from build123d import *

# Parameters (mm, degrees)
SKETCH1_W                       = 69.85
SKETCH1_H                       = 25.4
BASE_FLANGE1_DEPTH              = 4.55422
F_7_32_0_21875_DIAMETER_HOLE1_D = 5.55625
BREAK_CORNER1_DEPTH             = 4.55422
SKETCH4_W                       = 34.925
SKETCH4_H                       = 3.175
TAB1_DEPTH                      = 4.55422
FILLET1_R                       = 9.525
CUT_EXTRUDE1_REACH              = 40.633
SKETCH7_R                       = 9.525
CUT_EXTRUDE3_DEPTH              = 2.38125
F_9_32_0_28125_DIAMETER_HOLE1_D = 7.14375
FILLET3_R                       = 12.7
CUT_EXTRUDE4_START              = -2.17297
CUT_EXTRUDE4_DEPTH              = 2.17297
CUT_EXTRUDE5_REACH              = 40.633


# Read off the part's stored shape, not the designer's step: Break-Corner1
# Sheet-metal steps are written as plain solids
with BuildPart() as part:
    # Sketch1 → Base-Flange1 (new body)
    with BuildSketch(Plane.XY):
        Rectangle(SKETCH1_W, SKETCH1_H)
    extrude(amount=BASE_FLANGE1_DEPTH)

    # 7/32 (0.21875) Diameter Hole1 (through all)
    with Locations(Plane.XY.offset(4.55422)):
        with Locations((-28.575, 6.35), (-28.575, -6.35), (28.575, 6.35), (28.575, -6.35)):
            Hole(F_7_32_0_21875_DIAMETER_HOLE1_D / 2)

    # Break-Corner1 outline → Break-Corner1 (cut)
    with BuildSketch(Plane.XY):
        with BuildLine():
            Line((34.925, -12.7), (34.925, -9.525))
            ThreePointArc((34.925, -9.525), (33.99506403, -11.77006403), (31.75, -12.7))
            Line((31.75, -12.7), (34.925, -12.7))
        make_face()
        with BuildLine():
            ThreePointArc((31.75, 12.7), (33.99506403, 11.77006403), (34.925, 9.525))
            Line((34.925, 9.525), (34.925, 12.7))
            Line((34.925, 12.7), (31.75, 12.7))
        make_face()
        with BuildLine():
            Line((-34.925, -12.7), (-31.75, -12.7))
            ThreePointArc((-31.75, -12.7), (-33.99506403, -11.77006403), (-34.925, -9.525))
            Line((-34.925, -9.525), (-34.925, -12.7))
        make_face()
        with BuildLine():
            ThreePointArc((-34.925, 9.525), (-33.99506403, 11.77006403), (-31.75, 12.7))
            Line((-31.75, 12.7), (-34.925, 12.7))
            Line((-34.925, 12.7), (-34.925, 9.525))
        make_face()
    extrude(amount=BREAK_CORNER1_DEPTH, mode=Mode.SUBTRACT)

    # Sketch4 → Tab1 (add)
    with BuildSketch(Plane(origin=(0, 0, 0), x_dir=(-1, 0, 0), z_dir=(0, 0, -1))):
        with Locations((0, -14.2875)):
            Rectangle(SKETCH4_W, SKETCH4_H)
    extrude(amount=-TAB1_DEPTH)

    # Fillet1
    # the kernel refuses this fillet: 9.525 mm, written as the material it adds along each edge
    with BuildSketch(Plane(origin=(-17.4625, -12.7, 0), x_dir=(-1, 0, 0), z_dir=(0, 0, 1))) as fillet1_piece_1:
        with BuildLine():
            CenterArc((7.099515829, 9.525), FILLET1_R, 221.810314896, 48.189685104)
            Line((0, 3.175), (-0.141990317, 3.048))
            ThreePointArc((-0.141990317, 3.048), (-0.1905, 1.5875), (-0.1905, 0))
            Line((-0.1905, 0), (0, -0.1905))
            Line((0, -0.1905), (7.099515829, -0.1905))
            Line((7.099515829, -0.1905), (7.099515829, 0))
        make_face()
    extrude(amount=4.55422)
    with BuildSketch(Plane(origin=(17.4625, -12.7, 0), x_dir=(1, 0, 0), z_dir=(0, 0, 1))) as fillet1_piece_2:
        with BuildLine():
            CenterArc((7.099515829, -9.525), FILLET1_R, 90, 48.189685104)
            Line((0, -3.175), (-0.141990317, -3.048))
            ThreePointArc((-0.141990317, -3.048), (-0.1905, -1.5875), (-0.1905, 0))
            Line((-0.1905, 0), (0, 0.1905))
            Line((0, 0.1905), (7.099515829, 0.1905))
            Line((7.099515829, 0.1905), (7.099515829, 0))
        make_face()
    extrude(amount=4.55422)

    # Sketch5 → Cut-Extrude1 (cut, up to next)
    with BuildSketch(Plane(origin=(0, 0, 0), x_dir=(-1, 0, 0), z_dir=(0, 0, -1)), mode=Mode.PRIVATE) as cut_extrude1_sk1:
        with BuildLine():
            Line((-8.064231886, 9.525), (8.064231886, 9.525))
            ThreePointArc((8.064231886, 9.525), (9.864287689, 9.69663568), (11.599471303, 10.205357143))
            ThreePointArc((11.599471303, 10.205357143), (17.961811219, 12.070669174), (24.562015829, 12.7))
            Line((24.562015829, 12.7), (-24.562015829, 12.7))
            ThreePointArc((-24.562015829, 12.7), (-17.961811219, 12.070669174), (-11.599471303, 10.205357143))
            ThreePointArc((-11.599471303, 10.205357143), (-9.864287689, 9.69663568), (-8.064231886, 9.525))
        make_face()
    cut_extrude1_tool1 = extrude(cut_extrude1_sk1.sketch, amount=-CUT_EXTRUDE1_REACH, mode=Mode.PRIVATE) & part.part
    add(cut_extrude1_tool1.solids().sort_by_distance((0, 11.328032, 0))[0], mode=Mode.SUBTRACT)

    # Sketch7 → Cut-Extrude3 (cut)
    with BuildSketch(Plane(origin=(0, 0, 0), x_dir=(-1, 0, 0), z_dir=(0, 0, -1))):
        with Locations((0, -3.175)):
            Circle(SKETCH7_R)
    extrude(amount=-CUT_EXTRUDE3_DEPTH, mode=Mode.SUBTRACT)

    # 9/32 (0.28125) Diameter Hole1 (through all)
    with Locations(Plane(origin=(0, 0, 2.38125), x_dir=(-1, 0, 0), z_dir=(0, 0, -1))):
        with Locations((0, -3.175)):
            Hole(F_9_32_0_28125_DIAMETER_HOLE1_D / 2)

    # Fillet3
    fillet3_edges = [part.edges().sort_by_distance(p)[0] for p in [
        (17.4625, -15.875, 2.27711),
        (-17.4625, -15.875, 2.27711),
    ]]
    fillet(fillet3_edges, radius=FILLET3_R)

    # Sketch10 → Cut-Extrude4 (cut)
    with BuildSketch(Plane.XY.offset(4.55422).offset(CUT_EXTRUDE4_START)):
        with BuildLine():
            Line((3.571875, -2.38125), (3.571875, -5.55625))
            ThreePointArc((3.571875, -5.55625), (0, -9.128125), (-3.571875, -5.55625))
            Line((-3.571875, -5.55625), (-3.571875, -2.38125))
            ThreePointArc((-3.571875, -2.38125), (0, 1.190625), (3.571875, -2.38125))
        make_face()
    extrude(amount=CUT_EXTRUDE4_DEPTH, mode=Mode.SUBTRACT)

    # Sketch11 → Cut-Extrude5 (cut, up to next)
    with BuildSketch(Plane(origin=(0, 0, 0), x_dir=(-1, 0, 0), z_dir=(0, 0, -1)), mode=Mode.PRIVATE) as cut_extrude5_sk1:
        with BuildLine():
            Line((-22.225, -5.20921081), (-22.225, 4.475624183))
            ThreePointArc((-22.225, 4.475624183), (-21.675207986, 5.677006048), (-20.406646128, 6.046249135))
            ThreePointArc((-20.406646128, 6.046249135), (-17.13052876, 5.366731097), (-13.95629758, 4.308928571))
            ThreePointArc((-13.95629758, 4.308928571), (-13.839204583, 4.262663683), (-13.721748353, 4.217328884))
            ThreePointArc((-13.721748353, 4.217328884), (-12.980157851, 3.634624239), (-12.7, 2.734061773))
            Line((-12.7, 2.734061773), (-12.7, -7.790757838))
            ThreePointArc((-12.7, -7.790757838), (-13.312978112, -9.043939125), (-14.67853649, -9.329343784))
            ThreePointArc((-14.67853649, -9.329343784), (-15.557873342, -9.03604869), (-16.385140615, -8.617857143))
            ThreePointArc((-16.385140615, -8.617857143), (-18.616383766, -7.505452304), (-20.994274166, -6.756100736))
            ThreePointArc((-20.994274166, -6.756100736), (-21.879783228, -6.197587575), (-22.225, -5.20921081))
        make_face()
    cut_extrude5_tool1 = extrude(cut_extrude5_sk1.sketch, amount=-CUT_EXTRUDE5_REACH, mode=Mode.PRIVATE) & part.part
    cut_extrude5 = cut_extrude5_tool1.solids().sort_by_distance((17.387748, -1.405717, 0))[0]
    add(cut_extrude5, mode=Mode.SUBTRACT)

    # Mirror1: Cut-Extrude5 across plane
    add(cut_extrude5.mirror(Plane(origin=(0, 0, 0), x_dir=(0, 0, 1), z_dir=(1, 0, 0))), mode=Mode.SUBTRACT)


solid = part.part
Here's how the part is built. I have some questions about the finished solid (model axes, mm). A direction names the side the tool comes from. Round coordinates to 2 decimals unless told otherwise and drop trailing zeros. Loops run counter-clockwise (first coordinate to the right, second up) from the corner with the lowest first, then second, coordinate; pieces in that order, holes last. Notation, with made-up numbers: M -20,71.25 L -9,71.25 A21 ccw -9,97.25 Z; hole C 71.5,44.5 d10. An arc over 180 degrees is marked long. Write each question's results on one line, items separated by ' | '. Start each with the question number.
(1) Thinking about a two-plate mould opening in Y: for faces 1 (the cylindrical face through (-9.84, 9.69, 2.25)), 2 (the cylindrical face through (2.065, -12.473, 1.174)), 3 (the flat face through (12.7, -2, 2)), 4 (the flat face through (28, -12.7, 2)), which applies, pulls with the +Y half, pulls with the -Y half, needs draft (parallel to the pull), parting line crosses it, or undercut?
(2) I want a section at A-A (x = 0). Please give me the cut outline in (y, z) (3 decimals).
(3) Will these pins go through, and if not, where does the flat tip stop? P1, Ø4.5, axis at x = 28.575, y = -6.35, coming from the -Z side; P2, Ø9.5, axis at x = 2, y = -7, coming from the -Z side; P3, Ø2.5, axis at x = 1.5, z = 2.5, coming from the +Y side (3 decimals); P4, Ø1.4, axis at x = -29, z = 1.5, coming from the -Y side.
(4) I want a section at B-B (z = 3.45). State how many separate pieces and enclosed holes the cut face has, then the cut area to 3 significant figures.
(5) On a 3-axis mill with a long thin cutter (end or side, diameter ignored), from which of +Z, -Z, +X, -X, +Y, -Y can I reach the whole of each face in a straight line? I mean faces 5 (the flat face through (-4, -3, 2.381)), 6 (the flat face through (3.572, -4, 3)), 7 (the cylindrical face through (-34.02, 11.745, 2.245)). Say none if no direction works.
(6) If I drill on probe 1 along Y at (x, z) = (0, 1.5) (3 decimals); probe 2 along X at (y, z) = (-7.75, 3.6) (3 decimals); probe 3 along X at (y, z) = (8.25, 1.4) (3 decimals), over which ranges is the centre line in solid material (lowest first)? Write a range as from..to.
Solved:
1) face 1: pulls with the +Y half | face 2: undercut | face 3: undercut | face 4: pulls with the -Y half
2) outline: M -15.875,0 L -12.7,0 L -12.7,2.381 L -9.128,2.381 L -9.128,4.554 L -15.875,4.554 Z; M 1.191,2.381 L 6.35,2.381 L 6.35,0 L 9.525,0 L 9.525,4.554 L 1.191,4.554 Z
3) P1: passes through | P2: stops at z = 2.38 | P3: stops at y = 9.525 | P4: stops at y = -12.7
4) separate pieces: 1 | enclosed holes: 7 | area: 1,380 mm²
5) face 5: -Z | face 6: +Z, -Z | face 7: +Z, -Z, -X, +Y
6) probe 1: y = -15.875..-12.7, 6.35..9.525 | probe 2: x = -34.925..-30.975, -26.175..-18.044, -12.7..-2.819, 2.819..12.7, 18.044..26.175, 30.975..34.925 | probe 3: x = -34.925..-30.602, -26.548..26.548, 30.602..34.925
